```python
from build123d import *

# Parameters (mm, degrees)
SKETCH2_W           = 20
SKETCH2_H           = 40
BOSS_EXTRUDE2_DEPTH = 8
SKETCH3_R           = 2.1
CUT_EXTRUDE1_DEPTH  = 8
SKETCH4_R           = 1.5
CUT_EXTRUDE2_DEPTH  = 15


with BuildPart() as part:
    # Sketch2 → Boss-Extrude2 (new body)
    with BuildSketch(Plane(origin=(0, 33.757283518, 0), x_dir=(1, 0, 0), z_dir=(0, 1, 0))):
        with Locations((-80, 30.5)):
            Rectangle(SKETCH2_W, SKETCH2_H)
    extrude(amount=BOSS_EXTRUDE2_DEPTH)

    # Sketch3 → Cut-Extrude1 (cut)
    with BuildSketch(Plane(origin=(0, 41.757283518, 0), x_dir=(1, 0, 0), z_dir=(0, 1, 0))):
        with Locations(Location((-80, 15.5, 0), (0, 0, 270))):
            Circle(SKETCH3_R)
        with Locations(Location((-80, 45.5, 0), (0, 0, 270))):
            Circle(SKETCH3_R)
    extrude(amount=-CUT_EXTRUDE1_DEPTH, mode=Mode.SUBTRACT)

    # Sketch4 → Cut-Extrude2 (cut)
    with BuildSketch(Plane(origin=(-70, 0, 0), x_dir=(0, 0, -1), z_dir=(1, 0, 0))):
        with Locations(Location((25.5, 37.257283518, 0), (0, 0, 90))):
            Circle(SKETCH4_R)
        with Locations(Location((35.5, 37.257283518, 0), (0, 0, 90))):
            Circle(SKETCH4_R)
    extrude(amount=-CUT_EXTRUDE2_DEPTH, mode=Mode.SUBTRACT)


solid = part.part
```
The listing builds one solid part. Answer for the finished solid, in the listing's coordinates (mm). A direction names the side the tool comes from. Coordinates: 2 decimals unless noted, no trailing zeros. Write each loop counter-clockwise with the first axis right and the second up, starting at its lowest first coordinate (ties: lowest second). Pieces come first, ordered by that corner, then holes.
Q1. Section A-A, the plane x = -80 is taken. Write down the section's boundary in (y, z).
Returned:
outline: (33.76, -50.5) - (41.76, -50.5) - (41.76, -47.6) - (33.76, -47.6) - close; (33.76, -43.4) - (41.76, -43.4) - (41.76, -17.6) - (33.76, -17.6) - close; (33.76, -13.4) - (41.76, -13.4) - (41.76, -10.5) - (33.76, -10.5) - close; hole circle Ø3 at (37.26, -35.5); hole circle Ø3 at (37.26, -25.5)
Q2. The mould has two halves that part along Z. Classify faces 3 (the flat face through (-70, 38, -30)), 4 (the flat face through (-80, 38, -50.5)), 5 (the cylindrical face through (-80.8, 37.81, -43.56)): released by +Z, released by -Z, zero draft, split by the parting line, or undercut.
Returned:
face 3: zero draft
face 4: released by -Z
face 5: undercut
Q3. Section D-D, the plane z = -35.5 is taken. Write down the section's boundary in (x, y).
Returned:
outline: (-90, 33.76) - (-70, 33.76) - (-70, 35.76) - (-85, 35.76) - (-85, 38.76) - (-70, 38.76) - (-70, 41.76) - (-90, 41.76) - close
Q4. Find the intervals of material crossed by line 1 along Z through (x, y) = (-81.75, 35.25); line 2 along Z through (x, y) = (-78.75, 40.75); line 3 along Z through (x, y) = (-81.75, 36.75), in increasing order.
Returned:
line 1: z = -50.5 to -46.66, -44.34 to -16.66, -14.34 to -10.5
line 2: z = -50.5 to -47.19, -43.81 to -17.19, -13.81 to -10.5
line 3: z = -50.5 to -46.66, -44.34 to -36.91, -34.09 to -26.91, -24.09 to -16.66, -14.34 to -10.5
Q5. Section C-C, the plane y = 40 is taken. Write down the section's boundary in (x, z), then the cut area to 3 significant figures.
Returned:
outline: (-90, -50.5) - (-70, -50.5) - (-70, -10.5) - (-90, -10.5) - close; hole circle Ø4.2 at (-80, -45.5); hole circle Ø4.2 at (-80, -15.5)
area: 772 mm2
Q6. Given P1, Ø6.5, axis at x = -80, z = -15.5, coming from the +Y side; P2, Ø0.9, axis at y = 37, z = -25, coming from the +X side, each flat-ended and moving along its own axis, determine where each tip first touches the part or whether it passes through.
Returned:
P1: stops at y = 41.76
P2: stops at x = -85
Q7. Section B-B, the plane z = -45.5 is taken. Write down the section's boundary in (x, y), then the cut area to 3 significant figures.
Returned:
outline: (-90, 33.76) - (-82.1, 33.76) - (-82.1, 41.76) - (-90, 41.76) - close; (-77.9, 33.76) - (-70, 33.76) - (-70, 41.76) - (-77.9, 41.76) - close
area: 126 mm2
Q8. Which of the six approach directions +Z, -Z, +X, -X, +Y, -Y give full straight-line access (tool end or side, diameter ignored) to faces 1 (the flat face through (-85, 37, -25)), 2 (the flat face through (-80, 38, -10.5))?
Returned:
face 1: +X
face 2: +Z, +X, -X, +Y, -Y
